For this review, take the finished solid that the model builds, in its own axes (mm). A direction names the side the tool comes from. Round coordinates to 2 decimals unless told otherwise and drop trailing zeros. Write each loop counter-clockwise with the first axis right and the second up, starting at its lowest first coordinate (ties: lowest second). Pieces come first, ordered by that corner, then holes. Notation, with made-up numbers: (58.5, -29) -> (65.5, -29) arc R16 ccw to (65.5, -17) -> close; hole circle Ø5 at (-1, 28.5). An arc over 180 degrees is marked (long way). Write item = value, one per line. Start each with the question number.
Autodesk Inventor part; units mm, degrees
ref_plane "YZ Plane" through (0, 0, 0) normal (1, 0, 0) x (0, 1, 0)
ref_plane "XZ Plane" through (0, 0, 0) normal (0, 1, 0) x (-1, 0, 0)
ref_plane "XY Plane" through (0, 0, 0) normal (0, 0, 1) x (1, 0, 0)
sketch "Sketch1" plane through (0, 0, 0) normal (0, 1, 0) x (-1, 0, 0)
  line L0 (-29.924, 14.3694) -> (-29.924, -45.6306)
  line L1 (29.924, 14.3694) -> (29.924, -45.6306)
  line L2 (-7.574, -27.3788) -> (-7.574, -40.26)
  line L3 (-7.574, -40.26) -> (7.574, -40.26)
  line L4 (29.924, -45.6306) -> (-29.924, -45.6306)
  circle A0 centre (-23.749, 7.365) radius 1.5494
  arc A1 (23.749, 5.8156) -> (23.749, 8.9144) centre (23.749, 7.365) ccw
  circle A2 centre (10.414, -37.085) radius 1.5494
  line L5 (7.574, -33.91) -> (7.574, -40.26)
  circle A3 centre (23.6982, -25.782) radius 1.5494
  line L6 (7.574, -33.91) -> (18.924, -33.91)
  line L7 (-17.105, 14.3694) -> (-17.105, 3.065)
  line L8 (-22.624, 3.065) -> (-17.105, 3.065)
  line L9 (-22.624, 3.065) -> (-22.624, -27.3788)
  line L10 (-7.574, -27.3788) -> (-22.624, -27.3788)
  line L11 (18.924, -19.105) -> (18.924, -33.91)
  line L12 (18.924, -19.105) -> (24.424, -19.105)
  line L13 (23.749, -11.06) -> (24.424, -11.06)
  line L14 (24.424, -19.105) -> (24.424, -11.06)
  line L15 (-29.924, 14.3694) -> (-17.105, 14.3694)
  line L16 (22.1742, 14.3694) -> (29.924, 14.3694)
  line L17 (23.749, 5.8156) -> (23.7568, 5.8156)
  line L18 (23.749, 5.587) -> (23.749, -11.06)
  line L19 (22.1742, 14.3694) -> (22.1742, 8.9144)
  circle A4 centre (-10.414, -37.085) radius 1.5494
  line L20 (23.749, 5.587) -> (23.749, 5.8156)
  line L21 (23.749, 8.9144) -> (22.1742, 8.9144)
  point P0 (0, 0)
  point P1 (0, 0)
  dimension "d0" = 60
  dimension "d7" = 6.2258
  dimension "d8" = 19.8486
  dimension "d9" = 3.0988
  dimension "d12" = 12.8811
  dimension "d14" = 6.175
  dimension "d16" = 12.819
  dimension "d19" = 11
  dimension "d21" = 26.5256
  dimension "d22" = 34.5706
  dimension "d25" = 48.6956
  dimension "d27" = 5.5
  dimension "d28" = 6.175
  dimension "d30" = 7.3
  dimension "d31" = 11.7206
  dimension "d34" = 3.0988
  dimension "d35" = 3.0988
  dimension "d36" = 3.0988
  dimension "d38" = 8.5456
  dimension "d39" = 19.51
  dimension "d40" = 3.0988
  dimension "d41" = 8.5456
  dimension "d42" = 19.51
  dimension "d43" = 52.9956
  dimension "d44" = 6.175
  dimension "d176" = 5.455
  dimension "d177" = 7.7498
extrude "Extrusion1" add sketch "Sketch1" along normal blind 5.08 contours L15 L7 L8 L9 L10 L2 L3 L5 L6 L11 L12 L14 L13 L18 L20 A1 L21 L19 L16 L1 L4 L0 | A0 | A2 | A3 | A4
sketch "Sketch2" plane through (0, 0, 0) normal (0, -1, 0) x (1, 0, 0)
  line L0 (7.574, -40.26) -> (-7.574, -40.26)
  line L1 (-29.924, 14.3694) -> (-29.924, -45.6306)
  line L2 (-22.1742, 14.3694) -> (-29.924, 14.3694)
  line L3 (29.924, 14.3694) -> (17.105, 14.3694)
  line L4 (29.924, -45.6306) -> (29.924, 14.3694)
  line L5 (-26.924, 10.54) -> (26.924, 10.54)
  line L6 (-26.924, 10.54) -> (-26.924, -40.26)
  line L7 (-26.924, -40.26) -> (26.924, -40.26)
  line L8 (26.924, -40.26) -> (26.924, 10.54)
  point P0 (0, 0)
  dimension "d52" = 53.848
  dimension "d53" = 50.8
extrude "Extrusion3" cut sketch "Sketch2" against normal blind 0.7937
extrude "Extrusion2" cut sketch "Sketch1" along normal up to next contours A0 | A2 | A3 | A4
fillet "Fillet1" radius 5.08 4 edges at (29.924, 2.54, 14.3694) (29.924, 2.54, -45.6306) (-29.924, 2.54, -45.6306) (-29.924, 2.54, 14.3694)
fillet "Fillet2" radius 5.08 1 edges at (17.105, 2.54, 14.3694)
sketch "Sketch3" plane through (0, 0.7938, 0) normal (0, -1, 0) x (1, 0, 0)
  line L0 (-26.924, -40.26) -> (-26.924, 10.54)
  line L1 (-18.924, -33.91) -> (-7.574, -33.91)
  line L2 (-26.924, -40.26) -> (-14.224, -40.26)
  line L3 (-15.7226, -33.91) -> (-26.924, -33.91)
  line L4 (-26.924, -33.91) -> (-26.924, -40.26)
  line L5 (26.924, -40.26) -> (7.574, -40.26)
  line L6 (26.924, -40.26) -> (14.224, -40.26)
  line L7 (15.7226, -33.91) -> (26.924, -33.91)
  line L8 (26.924, -33.91) -> (26.924, -40.26)
  line L9 (-14.224, -40.26) -> (-14.224, -35.4086)
  line L10 (14.224, -40.26) -> (14.224, -35.4086)
  line L11 (14.224, -35.4086) -> (15.7226, -33.91)
  line L12 (-14.224, -35.4086) -> (-15.7226, -33.91)
  circle A0 centre (10.414, -37.085) radius 1.5494
  circle A1 centre (-10.414, -37.085) radius 1.5494
  point P0 (0, 0)
  dimension "d58" = 11.2014
  dimension "d59" = 11.2014
  dimension "d60" = 4.8514
  dimension "d61" = 4.8514
  dimension "d64" = 6.35
  dimension "d170" = 3.81
  dimension "d171" = 3.81
extrude "Extrusion4" add sketch "Sketch3" along normal blind 0.7937 contours L0 L3 L1 L12 L9 L2 | L5 L10 L11 L7 L8
sketch "Sketch4" plane through (0, 0, 0) normal (0, -1, 0) x (1, 0, 0)
  line L0 (0, -57.6306) -> (0, 26.3694)
  circle A0 centre (-21.3233, -39.7647) radius 1.5875
  line L1 (-15.7226, -33.91) -> (-26.924, -33.91)
  line L2 (-14.224, -40.26) -> (-14.224, -35.4086)
  circle A1 centre (21.3233, -39.7647) radius 1.5875
  dimension "d172" = 3.175
  dimension "d173" = 5.8547
  dimension "d174" = 7.0993
extrude "Extrusion5" cut sketch "Sketch4" against normal up to next
equation "\"d42\" = d39"
properties part number "back-cam"
1. Consider section B-B, the plane y = 4.1. Give the number of separate pieces and of enclosed holes in the cut face, then the cut area to 3 significant figures.
2. Consider section D-D, the plane z = 5. Give the boundary of the cut face in (x, y) (3 decimals).
3. Wall thickness on L1, parallel to X at y = 4.9, z = -29; L2, parallel to X at y = 1.75, z = -22.5; L3, parallel to X at y = 2.35, z = -26: over which ranges is each line inside the solid? List them lowest first. Write a range as from..to.
4. Draft analysis for pull direction Z (two halves, no side actions). For faces 5 (the flat face through (-23, 3, 8.914)), 6 (the cylindrical face through (28.48, 2.58, -44.1)), 7 (the flat face through (-21, 0, -37)), state which applies: +Z half, -Z half, draft (parallel to the pull), parting line (faces both ways), or undercut.
5. Consider section A-A, the plane z = -1. Give the boundary of the cut face in (x, y).
6. Clearance check with flat-ended pins moving along their axes: pin 1 Ø3 at (x, z) = (21.32, -39.76) entering from +Y; pin 2 Ø2 at (x, z) = (-21.5, -28) entering from -Y; pin 3 Ø10 at (x, z) = (5.5, -35) entering from +Y; pin 4 Ø3 at (x, y) = (-3, 3.5) entering from +Z. State where each tip first meets the part, or that it passes through.
7. Machinability: for faces 1 (the flat face through (-22, 3, -19.105)), 2 (the flat face through (20, 0, -37)), 3 (the flat face through (-14.96, 0.4, -34.67)), 4 (the flat face through (17.105, 3, 6)), which of the approach directions +Z, -Z, +X, -X, +Y, -Y give a long, thin tool a straight path to every point of the face, cutting with its end or side? Answer none if there is none.
Outcome:
q1.separate_pieces = 1
q1.enclosed_holes = 6
q1.area = 1,410 mm2
q2.outline = (-29.924, 0) -> (-26.924, 0) -> (-26.924, 0.794) -> (-23.749, 0.794) -> (-23.749, 5.08) -> (-29.924, 5.08) -> close; (17.105, 0.794) -> (26.924, 0.794) -> (26.924, 0) -> (29.924, 0) -> (29.924, 5.08) -> (17.105, 5.08) -> close
q3.L1 = -29.92..-18.92, 7.57..29.92
q3.L2 = -29.92..-18.92, 22.62..29.92
q3.L3 = -29.92..-25.23, -22.16..-18.92, 22.62..29.92
q4.face_5 = undercut
q4.face_6 = -Z half
q4.face_7 = draft
q5.outline = (-29.92, 0) -> (-26.92, 0) -> (-26.92, 0.79) -> (-23.75, 0.79) -> (-23.75, 5.08) -> (-29.92, 5.08) -> close; (22.62, 0.79) -> (26.92, 0.79) -> (26.92, 0) -> (29.92, 0) -> (29.92, 5.08) -> (22.62, 5.08) -> close
q6.pin_1 = through
q6.pin_2 = 0.79
q6.pin_3 = 5.08
q6.pin_4 = -40.26
q7.face_1 = +Y, -Y
q7.face_2 = +Z, -Z, +X, -X, -Y
q7.face_3 = +Z, -Y
q7.face_4 = +Z, +Y, -Y
